The listing builds one solid part. Answer for the finished solid, in the listing's coordinates (mm). Round coordinates to 2 decimals unless told otherwise and drop trailing zeros. Loops run counter-clockwise (first coordinate to the right, second up) from the corner with the lowest first, then second, coordinate; pieces in that order, holes last. Notation, with made-up numbers: M 9,80.5 L 50,80.5 A15 ccw 50,101.5 Z; hole C -24.75,15 d9. An arc over 180 degrees is marked long. Answer as a JSON object with one key per item and string values.
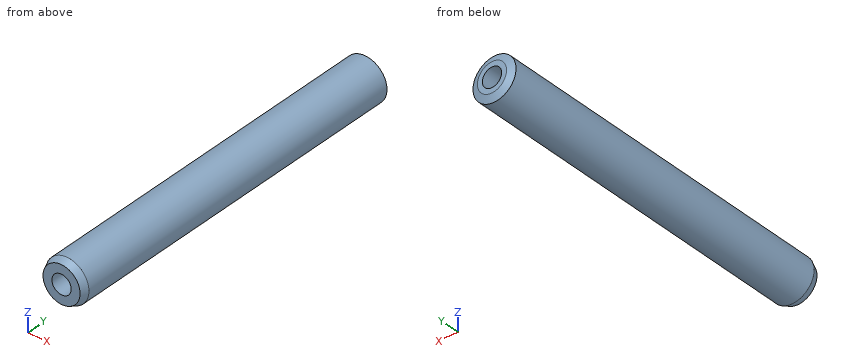
```python
from build123d import *
from OCP.BRepFilletAPI import BRepFilletAPI_MakeChamfer

# Parameters (mm, degrees)
SKETCH1_R           = 30
BOSS_EXTRUDE1_DEPTH = 501.286397
SKETCH2_R           = 13.435553616
CUT_EXTRUDE1_DEPTH  = 504.078574198
CHAMFER1_SIZE       = 9.678483
CHAMFER1_SIZE2      = 4.141442


with BuildPart() as part:
    # Sketch1 → Boss-Extrude1 (new body)
    with BuildSketch(Plane(origin=(0, 0, 0), x_dir=(1, 0, 0), z_dir=(0, 1, 0))):
        with Locations(Location((0, 0, 0), (0, 0, 270))):
            Circle(SKETCH1_R)
    extrude(amount=BOSS_EXTRUDE1_DEPTH)

    # Sketch2 → Cut-Extrude1 (cut, through all)
    with BuildSketch(Plane(origin=(0, 0, 0), x_dir=(1, 0, 0), z_dir=(0, 1, 0))):
        with Locations(Location((0, 0, 0), (0, 0, 270))):
            Circle(SKETCH2_R)
    extrude(amount=CUT_EXTRUDE1_DEPTH, mode=Mode.SUBTRACT)

    # Chamfer1: one chamfer whose edges measure the first distance from different faces: ONE call of the kernel's chamfer builder (chamfer() names one face for all edges)
    chamfer1_edges_1 = [part.edges().sort_by_distance(p)[0] for p in [
        (0, 0, -30),
    ]]
    chamfer1_side_1 = [part.faces().sort_by_distance(p)[0] for p in [
        (0, 250.6431985, -30),
    ]]
    chamfer1_edges_2 = [part.edges().sort_by_distance(p)[0] for p in [
        (0, 501.286397, -30),
    ]]
    chamfer1_side_2 = [part.faces().sort_by_distance(p)[0] for p in [
        (0, 501.286397, -29.151471863),
    ]]
    chamfer1 = BRepFilletAPI_MakeChamfer(part.part.solid().wrapped)
    for e in chamfer1_edges_1:
        chamfer1.Add(CHAMFER1_SIZE, CHAMFER1_SIZE2, e.wrapped, chamfer1_side_1[0].wrapped)  # the first distance lies on this face
    for e in chamfer1_edges_2:
        chamfer1.Add(CHAMFER1_SIZE, CHAMFER1_SIZE2, e.wrapped, chamfer1_side_2[0].wrapped)  # the first distance lies on this face
    add(Compound.cast(chamfer1.Shape()), mode=Mode.REPLACE)


solid = part.part
```
Item 1: The part is cut by section A-A (x = 0). Give the vertices of the cut face in (y, z), then the cut area to 3 significant figures.
Values follow:
{"outline": "M 0,-25.86 L 9.68,-30 L 497.14,-30 L 501.29,-20.32 L 501.29,-13.44 L 0,-13.44 Z; M 0,13.44 L 501.29,13.44 L 501.29,20.32 L 497.14,30 L 9.68,30 L 0,25.86 Z", "area": "16,500 mm^2"}
Item 2: Straight lines are drawn through the part: line 1 (X direction, y = 233.5, z = 0); line 2 (Z direction, x = -4.5, y = 161); line 3 (Z direction, x = 8, y = 208). For each, find the intervals that lie inside material, in ascending order.
Values follow:
{"line 1": "-30 to -13.44, 13.44 to 30", "line 2": "-29.66 to -12.66, 12.66 to 29.66", "line 3": "-28.91 to -10.79, 10.79 to 28.91"}
Item 3: The part is cut by section C-C (y = 361). Give the vertices of the cut face in (x, z), then the cut area to 3 significant figures.
Values follow:
{"outline": "C 0,0 d60; hole C 0,0 d26.87", "area": "2,260 mm^2"}
Item 4: Flat-ended cylindrical pins translate along their axes: P1, Ø6, axis at x = 7, y = 61, coming from the -Z side; P2, Ø2, axis at x = 14, y = 282.5, coming from the -Z side; P3, Ø10, axis at x = -20.5, y = 205.5, coming from the +Z side; P4, Ø24, axis at x = 0, z = 0, coming from the +Y side. Find the tip coordinate at first contact, or state that the pin passes through.
Values follow:
{"P1": "z = -29.73", "P2": "z = -27.04", "P3": "z = 25.69", "P4": "through"}
Item 5: The part is cut by section B-B (z = 0). Give the vertices of the cut face in (x, y), then the cut area to 3 significant figures.
Values follow:
{"outline": "M -30,9.68 L -25.86,0 L -13.44,0 L -13.44,501.29 L -20.32,501.29 L -30,497.14 Z; M 13.44,0 L 25.86,0 L 30,9.68 L 30,497.14 L 20.32,501.29 L 13.44,501.29 Z", "area": "16,500 mm^2"}
